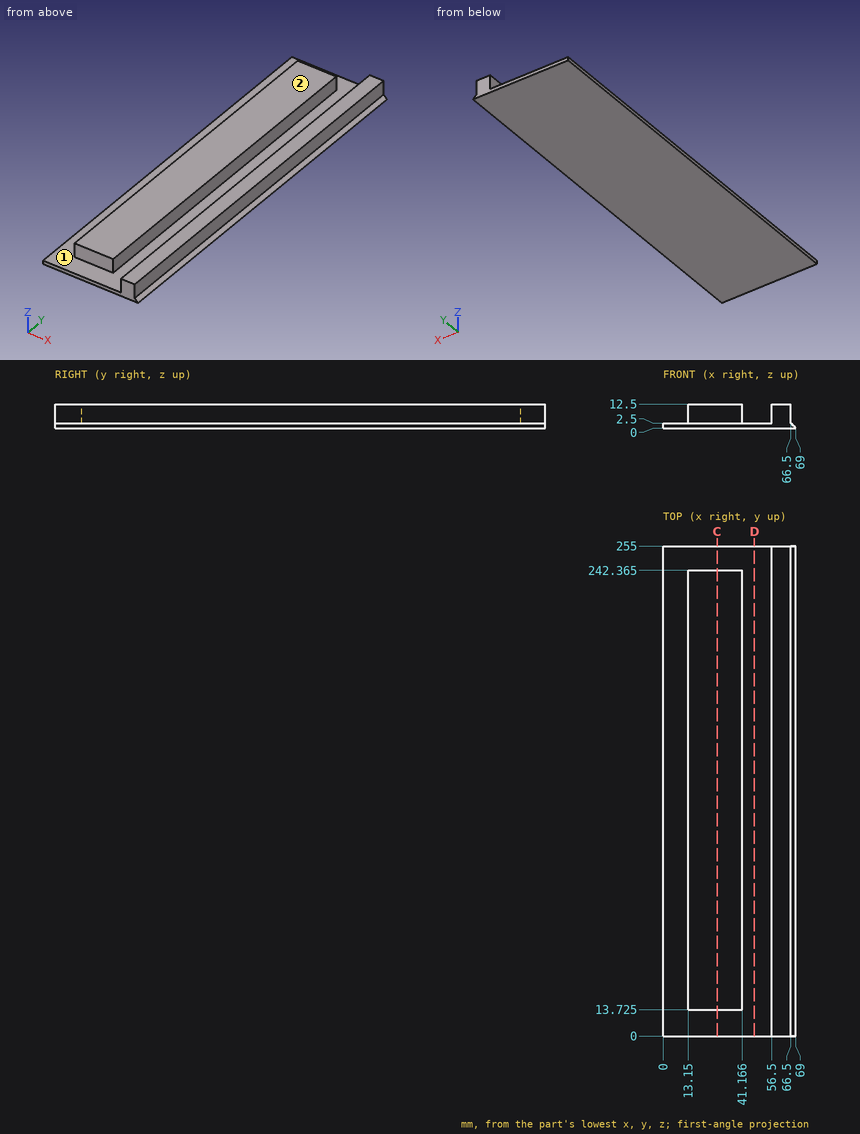
Here's the drawing with two shaded views (mm, measured from the low corner). I have some questions. Give positions to 0.01 mm unless a question says otherwise; leave off trailing zeros. Loops run counter-clockwise (first coordinate to the right, second up) from the corner with the lowest first, then second, coordinate; pieces in that order, holes last. Notation, with made-up numbers: (80.25, 68) -> (107.25, 68) arc R32 cw to (107.25, 103) -> close; hole circle Ø4 at (52, 77.5). An arc over 180 degrees is marked (long way). One line per item, written item: value.
Q1. I'm going to push flat-ended pins straight in: pin 1 Ø1.5 at (x, y) = (50, 194.5) entering from +Z; pin 2 Ø1 at (x, z) = (12.5, 11) entering from +Y; pin 3 Ø5 at (x, z) = (26, 6) entering from -Y (1 decimal); pin 4 Ø5 at (y, z) = (87.5, 9) entering from -X. Where does each tip first touch, or does it pass through?
Answers follow:
pin 1: z = 2.5
pin 2: through
pin 3: y = 13.7
pin 4: x = 13.15
Q2. If I drill on line 1 along Y through (x, z) = (39, 10.25) (1 decimal); line 2 along Z through (x, y) = (7, 178); line 3 along X through (y, z) = (93, 2), over which ranges is the centre line in solid material (lowest first)?
Answers follow:
line 1: 13.7 to 242.4
line 2: 0 to 2.5
line 3: 0 to 67
Q3. Suppose I cut it at D-D on x = 47.5. Please give me the cut outline in (y, z).
Answers follow:
outline: (0, 0) -> (255, 0) -> (255, 2.5) -> (0, 2.5) -> close
Q4. Suppose I cut it at C-C on x = 28. Please give me the cut outline in (y, z) (1 decimal), then the cut area to 3 significant figures.
Answers follow:
outline: (0, 0) -> (255, 0) -> (255, 2.5) -> (242.4, 2.5) -> (242.4, 12.5) -> (13.7, 12.5) -> (13.7, 2.5) -> (0, 2.5) -> close
area: 2,920 mm^2
Q5. We'd pull the mould along X, two halves only. Please class the marked faces 1 and 2: pulls with the +X half, pulls with the -X half, needs draft (parallel to the pull), parting line crosses it, or undercut.
Answers follow:
face 1: undercut
face 2: needs draft
